```python
from build123d import *

# Parameters (mm, degrees)
PAD_DEPTH       = 1.7
SKETCH004_W     = 15.98
SKETCH004_H     = 21.11
PAD007_DEPTH    = 13.45
POCKET008_DEPTH = 15


with BuildPart() as part:
    # Sketch → Pad (new body)
    with BuildSketch(Plane.XY):
        with BuildLine():
            Line((0, 0), (30, 0))
            Line((30, 0), (30, 1))
            Line((30, 1), (31, 1))
            Line((31, 1), (31, 18.27))
            Line((31, 18.27), (24.4, 18.27))
            ThreePointArc((24.4, 24.87), (21.1, 21.57), (24.4, 18.27))
            Line((24.4, 24.87), (31, 24.87))
            Line((31, 24.87), (31, 59.13))
            Line((31, 59.13), (24.4, 59.13))
            ThreePointArc((24.4, 65.73), (21.1, 62.43), (24.4, 59.13))
            Line((24.4, 65.73), (31, 65.73))
            Line((31, 65.73), (31, 83))
            Line((30, 83), (31, 83))
            Line((30, 84), (30, 83))
            Line((30, 84), (0, 84))
            Line((0, 84), (-30, 84))
            Line((-30, 84), (-30, 83))
            Line((-30, 83), (-31, 83))
            Line((-31, 83), (-31, 65.73))
            Line((-31, 65.73), (-24.4, 65.73))
            ThreePointArc((-24.4, 59.13), (-21.1, 62.43), (-24.4, 65.73))
            Line((-24.4, 59.13), (-31, 59.13))
            Line((-31, 59.13), (-31, 24.87))
            Line((-31, 24.87), (-24.4, 24.87))
            ThreePointArc((-24.4, 18.27), (-21.1, 21.57), (-24.4, 24.87))
            Line((-24.4, 18.27), (-31, 18.27))
            Line((-31, 18.27), (-31, 1))
            Line((-31, 1), (-30, 1))
            Line((-30, 1), (-30, 0))
            Line((-30, 0), (0, 0))
        make_face()
    extrude(amount=PAD_DEPTH)

    # Sketch004 → Pad007 (new body)
    with BuildSketch(Plane.XY.offset(1.7)):
        with Locations((18.935, 77.465)):
            Rectangle(SKETCH004_W, SKETCH004_H)
    extrude(amount=PAD007_DEPTH)

    # Sketch019 → Pocket008 (cut)
    with BuildSketch(Plane(origin=(0, 88.02, 0), x_dir=(-1, 0, 0), z_dir=(0, 1, 0))):
        Polygon((-24.825, 12.65), (-24.825, 5.72), (-21.915, 5.72), (-21.915, 4.02), (-20.97, 4.02), (-20.97, 2.6), (-16.9, 2.6), (-16.9, 4.02), (-15.955, 4.02), (-15.955, 5.72), (-13.045, 5.72), (-13.045, 12.65), align=None)
    extrude(amount=-POCKET008_DEPTH, mode=Mode.SUBTRACT)


solid = part.part
```
The listing builds one solid part. Answer for the finished solid, in the listing's coordinates (mm). A direction names the side the tool comes from. Coordinates: 2 decimals unless noted, no trailing zeros. Write each loop counter-clockwise with the first axis right and the second up, starting at its lowest first coordinate (ties: lowest second). Pieces come first, ordered by that corner, then holes. Notation, with made-up numbers: (18.25, 64) - (75.25, 64) arc R28 cw to (75.25, 85) - close; hole circle Ø1 at (64, 37). An arc over 180 degrees is marked (long way). Return JSON: item names as keys, results as strings. Group by question number.
1. Determine the mould class of faces 1 (the cylindrical face through (-21.1, 62.4, 0.8)), 2 (the flat face through (23, 81, 5.72)), 3 (the flat face through (19, 66.91, 8)) for opening direction X: released by +X, released by -X, zero draft, split by the parting line, or undercut.
2. A cutting plane is placed at C-C, the plane x = 15. Determine the outline of the cut face in (y, z), plus the area to 3 significant figures.
3. Given pin 1 (1.1 mm diameter, centred on x = 30.5, z = 1, fed in from +Y); pin 2 (7.5 mm diameter, centred on y = 77, z = 10, fed in from -X) (3 decimals); pin 3 (0.5 mm diameter, centred on x = -30.5, z = 0.5, fed in from +Y), each flat-ended and moving along its own axis, determine where each tip first touches the part or whether it passes through.
4. A cutting plane is placed at A-A, the plane y = 75.5. Determine the outline of the cut face in (x, z) (3 decimals), plus the area to 3 significant figures.
5. Which of the six approach directions +Z, -Z, +X, -X, +Y, -Y give full straight-line access (tool end or side, diameter ignored) to faces 4 (the flat face through (19, 86, 1.7)), 5 (the flat face through (-28, 18.27, 1)), 6 (the flat face through (21.915, 81, 5))?
6. A cutting plane is placed at D-D, the plane y = 45. Determine the outline of the cut face in (x, z).
7. A cutting plane is placed at B-B, the plane z = 11.25. Determine the outline of the cut face in (x, y) (3 decimals).
8. Straight lines are drawn through the part: L1, parallel to X at y = 74, z = 11.75 (3 decimals); L2, parallel to Z at x = -28, y = 27.5; L3, parallel to X at y = 70, z = 8.5 (3 decimals). For each, find the intervals that lie inside material, in ascending order.
Ans:
{
 "1": {"face 1": "released by -X", "face 2": "undercut", "face 3": "zero draft"},
 "2": {"outline": "(0, 0) - (84, 0) - (84, 1.7) - (88.02, 1.7) - (88.02, 5.72) - (73.02, 5.72) - (73.02, 12.65) - (88.02, 12.65) - (88.02, 15.15) - (66.91, 15.15) - (66.91, 1.7) - (0, 1.7) - close", "area": "323 mm²"},
 "3": {"pin 1": "y = 84", "pin 2": "x = 10.945", "pin 3": "y = 83"},
 "4": {"outline": "(-31, 0) - (31, 0) - (31, 1.7) - (26.925, 1.7) - (26.925, 15.15) - (10.945, 15.15) - (10.945, 1.7) - (-31, 1.7) - close; hole (13.045, 5.72) - (15.955, 5.72) - (15.955, 4.02) - (16.9, 4.02) - (16.9, 2.6) - (20.97, 2.6) - (20.97, 4.02) - (21.915, 4.02) - (21.915, 5.72) - (24.825, 5.72) - (24.825, 12.65) - (13.045, 12.65) - close", "area": "223 mm²"},
 "5": {"face 4": "-Z, +X, -X, +Y", "face 5": "+Z, -Z, -X", "face 6": "+Y"},
 "6": {"outline": "(-31, 0) - (31, 0) - (31, 1.7) - (-31, 1.7) - close"},
 "7": {"outline": "(10.945, 66.91) - (26.925, 66.91) - (26.925, 88.02) - (24.825, 88.02) - (24.825, 73.02) - (13.045, 73.02) - (13.045, 88.02) - (10.945, 88.02) - close"},
 "8": {"L1": "10.945 to 13.045, 24.825 to 26.925", "L2": "0 to 1.7", "L3": "10.945 to 26.925"}
}
